Source: CAD feature listing. Evaluate the final solid. Frame: model axes, mm. A direction names the side the tool comes from. Round coordinates to 2 decimals unless told otherwise and drop trailing zeros. Write each loop counter-clockwise with the first axis right and the second up, starting at its lowest first coordinate (ties: lowest second). Pieces come first, ordered by that corner, then holes.
```python
from build123d import *

# Parameters (mm, degrees)
F2_R     = 1.5875
F3_R     = 11.90625
F4_DEPTH = 27.78125
F5_R     = 3.96875
F6_DEPTH = 22.6893925511


with BuildPart() as f1:
    # F0 (on Right) → F1 (revolve)
    with BuildSketch(Plane.YZ):
        with BuildLine():
            Line((0, 128.5875), (0, 209.55))
            Line((0, 209.55), (-27.78125, 209.55))
            Line((-27.78125, 209.55), (-27.78125, 169.8879))
            Line((-27.78125, 169.8879), (-33.34385, 169.8879))
            Line((-33.34385, 169.8879), (-33.34385, 153.9875))
            Line((-33.34385, 153.9875), (-28.575, 153.9875))
            ThreePointArc((-28.575, 153.9875), (-24.0848719395, 152.1276280605), (-22.225, 147.6375))
            Line((-22.225, 147.6375), (-22.225, 111.76))
            Line((-22.225, 111.76), (-14.2875, 111.76))
            Line((-14.2875, 111.76), (-14.2875, 128.5875))
            Line((-14.2875, 128.5875), (0, 128.5875))
        make_face()
    revolve(axis=Axis((0, 90.567432344, 0), (0, 1, 0)))

    # F2
    f2_edges = [f1.edges().sort_by_distance(p)[0] for p in [
        (0, -27.78125, -169.8879),
    ]]
    fillet(f2_edges, radius=F2_R)

    # F3 (on face) → F4 (cut, through all)
    with BuildSketch(Plane(origin=(0, 0, 0), x_dir=(-1, 0, 0), z_dir=(0, 1, 0))):
        with Locations((0, 190.5)):
            Circle(F3_R)
        with Locations((-134.703841816, 134.703841816)):
            Circle(F3_R)
        with Locations((-190.5, 0)):
            Circle(F3_R)
        with Locations((-134.703841816, -134.703841816)):
            Circle(F3_R)
        with Locations((0, -190.5)):
            Circle(F3_R)
        with Locations((134.703841816, -134.703841816)):
            Circle(F3_R)
        with Locations((190.5, 0)):
            Circle(F3_R)
        with Locations((134.703841816, 134.703841816)):
            Circle(F3_R)
    extrude(amount=-F4_DEPTH, mode=Mode.SUBTRACT)

    # F5 (on face) → F6 (cut, through all)
    with BuildSketch(Plane(origin=(0, 0, 0), x_dir=(-1, 0, 0), z_dir=(0, 1, 0))):
        with Locations((0, 146.05)):
            Circle(F5_R)
        with Locations((-103.2729453923, 103.2729453923)):
            Circle(F5_R)
        with Locations((-146.05, 0)):
            Circle(F5_R)
        with Locations((-103.2729453923, -103.2729453923)):
            Circle(F5_R)
        with Locations((0, -146.05)):
            Circle(F5_R)
        with Locations((103.2729453923, -103.2729453923)):
            Circle(F5_R)
        with Locations((146.05, 0)):
            Circle(F5_R)
        with Locations((103.2729453923, 103.2729453923)):
            Circle(F5_R)
    extrude(amount=-F6_DEPTH, mode=Mode.SUBTRACT)


solid = f1.part
```
Q1. Section query A-A, the plane z = -190.5. Output: boundary loops of the cut face in (x, y).
Q2. Pin query (flat end, axial travel): P1, Ø14.5, axis at x = 0, z = -190.5, coming from the +Y side; P2, Ø4, axis at x = -163, y = -29, coming from the +Z side; P3, Ø6, axis at y = -28.5, z = -153, coming from the +X side; P4, Ø3, axis at x = -148.5, y = -28, coming from the +Z side. Return the tip coordinate at first contact, or that it passes through.
Q3. Section query B-B, the plane y = -8. Give the number of separate pieces and of enclosed holes in the cut face, and give its area (3 significant figures).
Q4. Section query C-C, the plane x = 190.5. Output: boundary loops of the cut face in (y, z), and give its area (3 significant figures).
Q5. Line query: line 1 (Y direction, x = -125, z = -123); line 2 (X direction, y = -26.5, z = -126); line 3 (Z direction, x = -191, y = -23.5). Output: solid intervals per line, ascending.
Q6. Set-up query: faces 1 (the face through (-201.856, -13.696, 3.576)), 2 (the face through (172, -27.781, -1)), 3 (the face through (-78.243, -7.044, -102.043)). Return all of +Z, -Z, +X, -X, +Y, -Y with unobstructed straight access to the full face (end or side cutting, diameter ignored); none if empty.
Q7. Mould query, pull axis X, two halves, no side actions, for faces 4 (the face through (3, 0, -137)), 5 (the face through (105, -14.287, 39)), 6 (the face through (-204.567, -14.085, -45.426)). Classes: pulls with the +X half, pulls with the -X half, needs draft (parallel to the pull), parting line crosses it, or undercut.
Filled in:
1. outline: (-87.3, -27.78) - (-11.91, -27.78) - (-11.91, 0) - (-87.3, 0) - close; (11.91, -27.78) - (87.3, -27.78) - (87.3, 0) - (11.91, 0) - close
2. P1: passes through
2. P2: stops at z = 133.63
2. P3: stops at x = 146.24
2. P4: stops at z = 149.32
3. separate pieces: 1
3. enclosed holes: 17
3. area: 82,000 mm2
4. outline: (-27.78, -87.3) - (0, -87.3) - (0, -11.91) - (-27.78, -11.91) - close; (-27.78, 11.91) - (0, 11.91) - (0, 87.3) - (-27.78, 87.3) - close
4. area: 4,190 mm2
5. line 1: y = -27.78 to 0
5. line 2: x = -167.44 to -142.83, -126.58 to -87.91, 87.91 to 126.58, 142.83 to 167.44
5. line 3: z = -86.2 to -11.9, 11.9 to 86.2
6. face 1: +Y, -Y
6. face 2: -Y
6. face 3: +Y
7. face 4: needs draft
7. face 5: undercut
7. face 6: parting line crosses it
